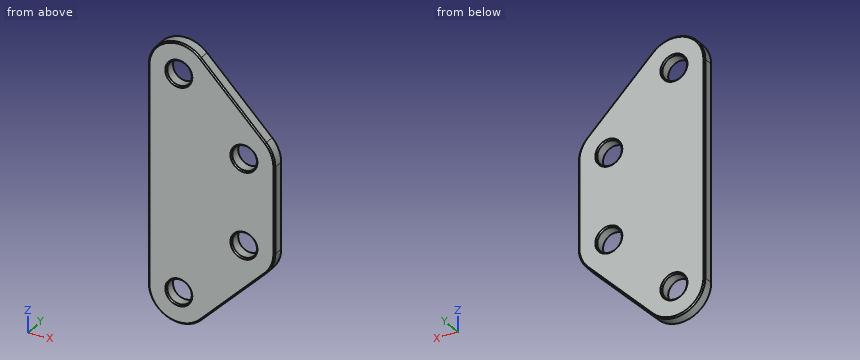
```python
from build123d import *

# Parameters (mm, degrees)
SKETCH1_R           = 20
BOSS_EXTRUDE1_DEPTH = 20
CHAMFER1_SIZE       = 2


with BuildPart() as part:
    # Sketch1 → Boss-Extrude1 (new body)
    with BuildSketch(Plane(origin=(0, 0, 0), x_dir=(1, 0, 0), z_dir=(0, 1, 0))):
        with BuildLine():
            Line((-100, 176.066017178), (-100, -176.066017178))
            ThreePointArc((-100, -176.066017178), (-69.134171618, -222.259993804), (-14.644660941, -211.421356237))
            Line((-14.644660941, -211.421356237), (91.421356237, -105.355339059))
            ThreePointArc((91.421356237, -105.355339059), (102.259993804, -89.134171618), (106.066017178, -70))
            Line((106.066017178, -70), (106.066017178, 70))
            ThreePointArc((106.066017178, 70), (102.259993804, 89.134171618), (91.421356237, 105.355339059))
            Line((91.421356237, 105.355339059), (-14.644660941, 211.421356237))
            ThreePointArc((-14.644660941, 211.421356237), (-69.134171618, 222.259993804), (-100, 176.066017178))
        make_face()
        with Locations(Location((-50, 176.066017178, 0), (0, 0, 270))):
            Circle(SKETCH1_R, mode=Mode.SUBTRACT)
        with Locations(Location((56.066017178, 70, 0), (0, 0, 270))):
            Circle(SKETCH1_R, mode=Mode.SUBTRACT)
        with Locations(Location((56.066017178, -70, 0), (0, 0, 270))):
            Circle(SKETCH1_R, mode=Mode.SUBTRACT)
        with Locations(Location((-50, -176.066017178, 0), (0, 0, 270))):
            Circle(SKETCH1_R, mode=Mode.SUBTRACT)
    extrude(amount=BOSS_EXTRUDE1_DEPTH)

    # Chamfer1
    chamfer1_edges = [part.edges().sort_by_distance(p)[0] for p in [
        (106.066017178, 0, 0),
        (102.259993804, 0, 89.134171618),
        (38.388347648, 0, 158.388347648),
        (-69.134171618, 0, 222.259993804),
        (102.259993804, 20, 89.134171618),
        (106.066017178, 20, 0),
        (102.259993804, 20, -89.134171618),
        (-50, 0, -196.066017178),
        (-50, 20, -196.066017178),
        (38.388347648, 20, -158.388347648),
        (56.066017178, 0, -90),
        (56.066017178, 20, -90),
        (-69.134171618, 20, -222.259993804),
        (56.066017178, 0, 50),
        (56.066017178, 20, 50),
        (-100, 20, 0),
        (-50, 0, 156.066017178),
        (-50, 20, 156.066017178),
        (-69.134171618, 20, 222.259993804),
        (-100, 0, 0),
        (38.388347648, 20, 158.388347648),
        (-69.134171618, 0, -222.259993804),
        (38.388347648, 0, -158.388347648),
        (102.259993804, 0, -89.134171618),
    ]]
    chamfer(chamfer1_edges, length=CHAMFER1_SIZE)


solid = part.part
```
For this review, take the finished solid that the model builds, in its own axes (mm). Round coordinates to 2 decimals unless told otherwise and drop trailing zeros. Write each loop counter-clockwise with the first axis right and the second up, starting at its lowest first coordinate (ties: lowest second). Pieces come first, ordered by that corner, then holes. Notation, with made-up numbers: (-20.75, 9.25) -> (-2.75, 9.25) arc R11 cw to (-2.75, 23.25) -> close; hole circle Ø4 at (-2, 82.25). An arc over 180 degrees is marked (long way). Use one line per item in the form item = value.
Q1. Consider section A-A (x = -50). State the section outline as (y, z) points, then the cut area to 3 significant figures.
Resolved:
outline = (0, -224.07) -> (2, -226.07) -> (18, -226.07) -> (20, -224.07) -> (20, -198.07) -> (18, -196.07) -> (2, -196.07) -> (0, -198.07) -> close; (0, -154.07) -> (2, -156.07) -> (18, -156.07) -> (20, -154.07) -> (20, 154.07) -> (18, 156.07) -> (2, 156.07) -> (0, 154.07) -> close; (0, 198.07) -> (2, 196.07) -> (18, 196.07) -> (20, 198.07) -> (20, 224.07) -> (18, 226.07) -> (2, 226.07) -> (0, 224.07) -> close
area = 7,420 mm²
Q2. Consider section C-C (z = -140). State the section outline as (x, y) points.
Resolved:
outline = (-100, 2) -> (-98, 0) -> (53.95, 0) -> (56.78, 2) -> (56.78, 18) -> (53.95, 20) -> (-98, 20) -> (-100, 18) -> close
Q3. Clearance check with flat-ended pins moving along their axes: pin 1 Ø4 at (x, y) = (50.5, 6) entering from -Z; pin 2 Ø6 at (x, y) = (80, 8.5) entering from +Z; pin 3 Ø1.5 at (x, y) = (71.5, 5) entering from -Z. State where each tip first meets the part, or that it passes through.
Resolved:
pin_1 = -148.28
pin_2 = 119.78
pin_3 = -126.03
Q4. Consider section B-B (y = 6). State the section outline as (x, z) points.
Resolved:
outline = (-100, -176.07) arc R50 ccw to (-14.64, -211.42) -> (91.42, -105.36) arc R50 ccw to (106.07, -70) -> (106.07, 70) arc R50 ccw to (91.42, 105.36) -> (-14.64, 211.42) arc R50 ccw to (-100, 176.07) -> close; hole circle Ø40 at (-50, -176.07); hole circle Ø40 at (-50, 176.07); hole circle Ø40 at (56.07, -70); hole circle Ø40 at (56.07, 70)
Q5. Consider section D-D (x = 49). State how many separate pieces and enclosed holes the cut face has, then the cut area to 3 significant figures.
Resolved:
separate_pieces = 3
enclosed_holes = 0
area = 4,390 mm²
Q6. To check wall thickness, follow probe 1 along Z at (x, y) = (-54, 19); probe 2 along Z at (x, y) = (42, 5.5); probe 3 along X at (y, z) = (8.5, -70). State the ranges of each line that lie inside material, in increasing order. Write a range as from..to.
Resolved:
probe_1 = -224.9..-196.68, -155.45..155.45, 196.68..224.9
probe_2 = -154.78..-84.22, -55.78..55.78, 84.22..154.78
probe_3 = -100..36.07, 76.07..106.07
